Answer from the drawing. Dimensions are ordinates in mm from the lowest x, y and z of the part. A direction names the side the tool comes from. Coordinates: 2 decimals unless noted, no trailing zeros. Write each loop counter-clockwise with the first axis right and the second up, starting at its lowest first coordinate (ties: lowest second). Pieces come first, ordered by that corner, then holes.
(1) Which of the six approach directions +Z, -Z, +X, -X, +Y, -Y give full straight-line access (tool end or side, diameter ignored) to the marked faces 4 and 5?
(2) Section D-D on x = 8.25 is taken. Write down the section's boundary in (y, z) (1 decimal).
(3) Section B-B on y = 7 is taken. Write down the section's boundary in (x, z).
(4) Section A-A on x = 4.75 is taken. Write down the section's boundary in (y, z) (1 decimal).
(5) Find the intervals of material crossed by probe 1 along X at (y, z) = (5.5, 5) (1 decimal); probe 2 along Z at (x, y) = (8.5, 2.5), in increasing order.
(6) Section C-C on y = 2.25 is taken. Write down the section's boundary in (x, z).
(7) Given pin 1 (1.5 mm diameter, centred on y = 2, z = 7, fed in from -X); pin 2 (6 mm diameter, centred on x = 1.5, z = 4.5, fed in from -Y); pin 3 (1.5 mm diameter, centred on y = 4, z = 9, fed in from +X), each flat-ended and moving along its own axis, determine where each tip first touches the part or whether it passes through.
(8) The mould has two halves that part along Y. Classify the marked faces 1, 2 and 3: +Y half, -Y half, draft (parallel to the pull), parting line (faces both ways), or undercut.
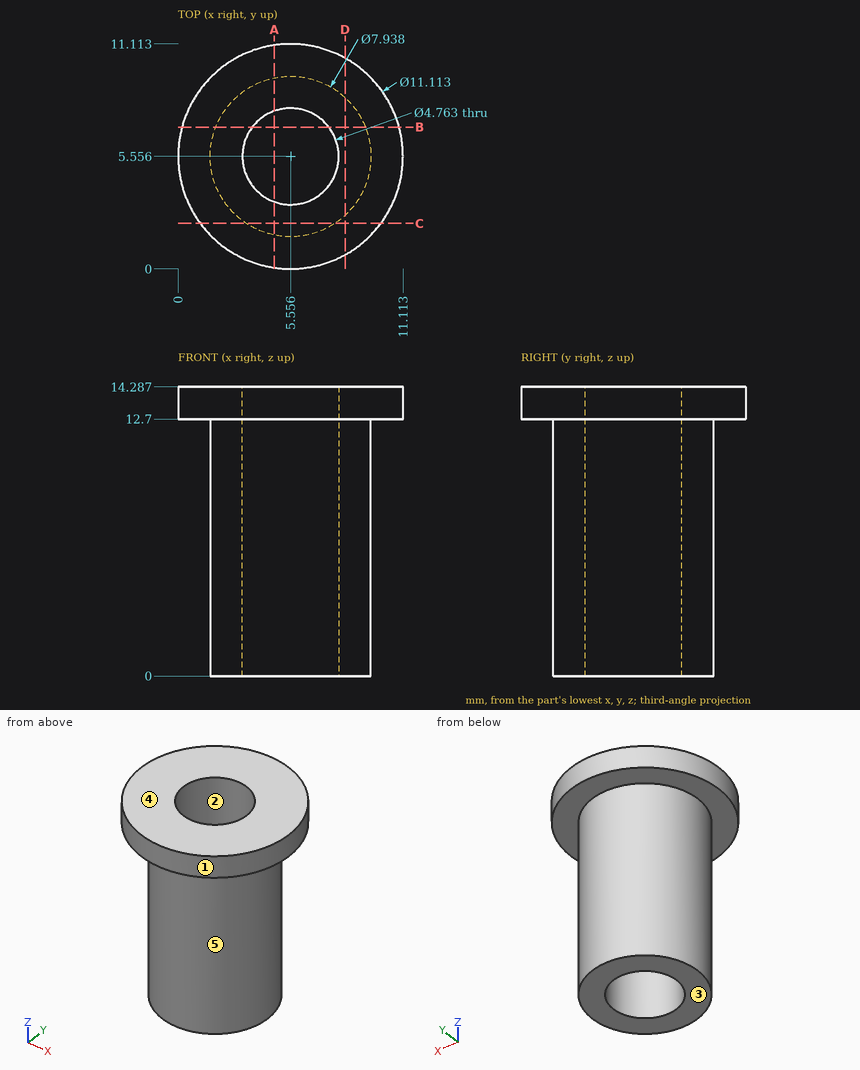
Response:
1. face 4: +Z, +X, -X, +Y, -Y
1. face 5: -Z
2. outline: (0.7, 12.7) - (2.6, 12.7) - (2.6, 0) - (8.5, 0) - (8.5, 12.7) - (10.4, 12.7) - (10.4, 14.3) - (0.7, 14.3) - close
3. outline: (0.19, 12.7) - (1.86, 12.7) - (1.86, 0) - (3.66, 0) - (3.66, 14.29) - (0.19, 14.29) - close; (7.45, 0) - (9.25, 0) - (9.25, 12.7) - (10.92, 12.7) - (10.92, 14.29) - (7.45, 14.29) - close
4. outline: (0.1, 12.7) - (1.7, 12.7) - (1.7, 0) - (3.3, 0) - (3.3, 14.3) - (0.1, 14.3) - close; (7.8, 0) - (9.4, 0) - (9.4, 12.7) - (11.1, 12.7) - (11.1, 14.3) - (7.8, 14.3) - close
5. probe 1: x = 1.6 to 3.2, 7.9 to 9.5
5. probe 2: z = 12.7 to 14.29
6. outline: (1.09, 12.7) - (3.36, 12.7) - (3.36, 0) - (7.75, 0) - (7.75, 12.7) - (10.02, 12.7) - (10.02, 14.29) - (1.09, 14.29) - close
7. pin 1: stops at x = 2.75
7. pin 2: stops at y = 1.73
7. pin 3: stops at x = 9.44
8. face 1: parting line
8. face 2: undercut
8. face 3: draft
